Verification items for the finished model (mm, model axes). A direction names the side the tool comes from. Give positions to 0.01 mm unless a question says otherwise; leave off trailing zeros. Write each loop counter-clockwise with the first axis right and the second up, starting at its lowest first coordinate (ties: lowest second). Pieces come first, ordered by that corner, then holes. Notation, with made-up numbers: M 86.25,-35 L 100.25,-35 A5 ccw 100.25,-26 Z; hole C -4,22 d1. An arc over 180 degrees is marked long. Answer as a JSON object with one key per item and string values.
```python
from build123d import *

# Parameters (mm, degrees)
EXTRUDE_1_DEPTH     = 65
SKETCH_4_R          = 2.25
CUT_EXTRUDE_2_DEPTH = 44
CUT_EXTRUDE_START   = -3
SKETCH_5_R          = 3.75
CUT_EXTRUDE_3_DEPTH = 44
EXTRUDE_2_DEPTH     = 5
EXTRUDE_3_DEPTH     = 8
SKETCH_8_R          = 2.3
CUT_EXTRUDE_4_DEPTH = 3.5
CUT_EXTRUDE_6_DEPTH = 14
CUT_EXTRUDE_7_DEPTH = 5


with BuildPart() as part:
    # ｽｹｯﾁ1 → ﾎﾞｽ - 押し出し1 (new body)
    with BuildSketch(Plane.XY):
        Polygon((0, 0), (5.13030215, 14.095389312), (-8.965087162, 19.225691462), (-7.254986445, 23.924154566), (53.707680142, 23.924154566), (53.707680142, 18.924154566), (4.698463104, -1.710100717), align=None)
    extrude(amount=EXTRUDE_1_DEPTH)

    # ｽｹｯﾁ4 → ｶｯﾄ - 押し出し2 (cut)
    with BuildSketch(Plane(origin=(5.13030215, 14.095389312, 0), x_dir=(-0.939692621, 0.342020143, 0), z_dir=(-0.342020143, -0.939692621, 0))):
        with Locations((7.5, -7.5)):
            Circle(SKETCH_4_R)
        with Locations((7.5, -52.5)):
            Circle(SKETCH_4_R)
    extrude(amount=-CUT_EXTRUDE_2_DEPTH, mode=Mode.SUBTRACT)

    # ｽｹｯﾁ5 → ｶｯﾄ - 押し出し3 (cut)
    with BuildSketch(Plane(origin=(5.13030215, 14.095389312, 0), x_dir=(-0.939692621, 0.342020143, 0), z_dir=(-0.342020143, -0.939692621, 0)).offset(CUT_EXTRUDE_START)):
        with Locations((7.5, -52.5)):
            Circle(SKETCH_5_R)
        with Locations((7.5, -7.5)):
            Circle(SKETCH_5_R)
    extrude(amount=-CUT_EXTRUDE_3_DEPTH, mode=Mode.SUBTRACT)

    # ｽｹｯﾁ6 → ﾎﾞｽ - 押し出し2 (add)
    with BuildSketch(Plane(origin=(0, 0, 65), x_dir=(-1, 0, 0), z_dir=(0, 0, -1))):
        Polygon((-53.707680142, 33.124154566), (-53.707680142, 18.924154566), (-4.698463104, -1.710100717), (0, 0), (-5.13030215, 14.095389312), (8.965087162, 19.225691462), (3.90646029, 33.124154566), align=None)
    extrude(amount=-EXTRUDE_2_DEPTH)

    # ｽｹｯﾁ7 → ﾎﾞｽ - 押し出し3 (add)
    with BuildSketch(Plane(origin=(0, 0, 65), x_dir=(-1, 0, 0), z_dir=(0, 0, -1))):
        Polygon((3.90646029, 33.124154566), (5.726311461, 28.124154566), (-53.707680142, 28.124154566), (-53.707680142, 33.124154566), align=None)
    extrude(amount=EXTRUDE_3_DEPTH)

    # ｽｹｯﾁ8 → ｶｯﾄ - 押し出し4 (cut)
    with BuildSketch(Plane(origin=(0, 23.924154566, 0), x_dir=(1, 0, 0), z_dir=(0, 1, 0))):
        with Locations((7.695013555, -30)):
            Circle(SKETCH_8_R)
    extrude(amount=-CUT_EXTRUDE_4_DEPTH, mode=Mode.SUBTRACT)

    # ｽｹｯﾁ10 → ｶｯﾄ - 押し出し6 (cut, through all)
    with BuildSketch(Plane(origin=(0, 0, 57), x_dir=(-1, 0, 0), z_dir=(0, 0, -1))):
        Polygon((7.254986445, 23.924154566), (-11.09353971, 23.924154566), (-11.09353971, 33.124154566), (3.90646029, 33.124154566), align=None)
    extrude(amount=-CUT_EXTRUDE_6_DEPTH, mode=Mode.SUBTRACT)

    # ｽｹｯﾁ11 → ｶｯﾄ - 押し出し7 (cut)
    with BuildSketch(Plane(origin=(53.707680142, 0, 0), x_dir=(0, 0, -1), z_dir=(1, 0, 0))):
        Polygon((-65, 23.924154566), (-70, 23.924154566), (-70, 33.124154566), (-57, 33.124154566), (-57, 28.124154566), (-65, 28.124154566), align=None)
    extrude(amount=-CUT_EXTRUDE_7_DEPTH, mode=Mode.SUBTRACT)


solid = part.part
```
1) Section check C-C on z = 17. Record the boundary of the cut face in (x, y), and give its area (3 significant figures).
Completed:
{"outline": "M -8.97,19.23 L 5.13,14.1 L 0,0 L 4.7,-1.71 L 53.71,18.92 L 53.71,23.92 L -7.25,23.92 Z", "area": "879 mm2"}
2) Section check B-B on x = 22. Record the boundary of the cut face in (y, z), and give its area (3 significant figures).
Completed:
{"outline": "M 5.57,0 L 23.92,0 L 23.92,65 L 28.12,65 L 28.12,57 L 33.12,57 L 33.12,70 L 5.57,70 Z", "area": "1,370 mm2"}
3) Go/stop test with flat-tipped pins: pin 1 (4.5 mm diameter, centred on y = 30, z = 62, fed in from +X); pin 2 (12 mm diameter, centred on x = 34.5, z = 38, fed in from +Y); pin 3 (1 mm diameter, centred on y = 8, z = 22.5, fed in from +X). Record where each tip stops, or that it passes through.
Completed:
{"pin 1": "stops at x = 48.71", "pin 2": "stops at y = 23.92", "pin 3": "stops at x = 28.95"}
4) Release check for a two-part mould opening along Y. For faces 1 (the face through (11.094, 29, 65)), 2 (the face through (30, 28.124, 61)), 3 (the face through (-3.191, 20.317, 52.448)), 4 (the face through (2.382, -0.867, 34.51)) record: pulls with the +Y half, pulls with the -Y half, needs draft (parallel to the pull), parting line crosses it, or undercut.
Completed:
{"face 1": "needs draft", "face 2": "undercut", "face 3": "undercut", "face 4": "pulls with the -Y half"}
5) Section check A-A on z = 30. Record the boundary of the cut face in (x, y).
Completed:
{"outline": "M -8.97,19.23 L 5.13,14.1 L 0,0 L 4.7,-1.71 L 53.71,18.92 L 53.71,23.92 L 10,23.92 L 10,20.42 L 5.4,20.42 L 5.4,23.92 L -7.25,23.92 Z"}
6) Access from +Z, -Z, +X, -X, +Y, -Y to the whole of each face (thin tool, end or side, straight path). Record for faces 5 (the face through (8, 20.424, 30)), 6 (the face through (2.53, 6.95, 34.51)), 7 (the face through (30, 26, 65)), 8 (the face through (30, 31, 57)), 9 (the face through (48.708, 30, 65)).
Completed:
{"face 5": "+Y", "face 6": "+Z, -Z, -X", "face 7": "-Z, +X, -X", "face 8": "-Z, +X, -X, +Y", "face 9": "+Z, -Z, +X, +Y"}
7) Thickness scan on L1, parallel to Z at x = 33, y = 30; L2, parallel to X at y = 22.7, z = 30; L3, parallel to X at y = 21, z = 30. Record the ranges inside material, lowest first.
Completed:
{"L1": "z = 57 to 70", "L2": "x = -7.7 to 5.4, 10 to 53.71", "L3": "x = -8.32 to 5.4, 10 to 53.71"}
8) Section check D-D on y = 9. Record the boundary of the cut face in (x, z).
Completed:
{"outline": "M 3.28,0 L 30.14,0 L 30.14,70 L 3.28,70 Z"}
